```python
from build123d import *

# Parameters (mm, degrees)
SKETCH_1_R          = 3
EXTRUDE_1_DEPTH     = 1
SKETCH_2_R          = 2.5
EXTRUDE_2_DEPTH     = 7.6
FILLET_1_R          = 2.5
SKETCH_4_R          = 2.556662668
CUT_EXTRUDE_1_DEPTH = 1.1


with BuildPart() as part:
    # Эскиз1 → Бобышка-Вытянуть1 (new body)
    with BuildSketch(Plane(origin=(0, 0, 0), x_dir=(1, 0, 0), z_dir=(0, 1, 0))):
        with Locations(Location((0, 0, 0), (0, 0, 270))):
            Circle(SKETCH_1_R)
    extrude(amount=EXTRUDE_1_DEPTH)

    # Эскиз2 → Бобышка-Вытянуть2 (add)
    with BuildSketch(Plane(origin=(0, 1, 0), x_dir=(1, 0, 0), z_dir=(0, 1, 0))):
        with Locations(Location((0, 0, 0), (0, 0, 90))):
            Circle(SKETCH_2_R)
    extrude(amount=EXTRUDE_2_DEPTH)

    # Скругление1
    fillet_1_edges = [part.edges().sort_by_distance(p)[0] for p in [
        (0, 8.6, 2.5),
    ]]
    fillet(fillet_1_edges, radius=FILLET_1_R)

    # Эскиз4 → Вырез-Вытянуть1 (cut)
    with BuildSketch(Plane(origin=(0, 8.6, 0), x_dir=(1, 0, 0), z_dir=(0, 1, 0))):
        Circle(SKETCH_4_R)
    extrude(amount=-CUT_EXTRUDE_1_DEPTH, mode=Mode.SUBTRACT)


solid = part.part
```
For this review, take the finished solid that the model builds, in its own axes (mm). A direction names the side the tool comes from. Round coordinates to 2 decimals unless told otherwise and drop trailing zeros. Write each loop counter-clockwise with the first axis right and the second up, starting at its lowest first coordinate (ties: lowest second). Pieces come first, ordered by that corner, then holes. Notation, with made-up numbers: (43, 3) - (88, 3) arc R13 cw to (88, 26) - close; hole circle Ø9 at (-13, -26.75). An arc over 180 degrees is marked (long way). Answer as a JSON object with one key per item and string values.
1. We need section C-C on y = 2.25. Give the boundary of the cut face in (x, z).
Response values:
{"outline": "circle Ø5 at (0, 0)"}
2. For pin 1 Ø1 at (x, y) = (-1, 6.5) entering from +Z; pin 2 Ø1 at (y, z) = (2.5, 0) entering from +X; pin 3 Ø2 at (x, y) = (2, 4) entering from -Z, all flat-tipped, find the tip position at first contact; note any pin that passes through.
Response values:
{"pin 1": "stops at z = 2.43", "pin 2": "stops at x = 2.5", "pin 3": "stops at z = -2.29"}
3. To check wall thickness, follow line 1 along Y through (x, z) = (-2.3, 1.85); line 2 along Z through (x, y) = (0.05, 2). State the ranges of each line that lie inside material, in increasing order.
Response values:
{"line 1": "y = 0 to 1", "line 2": "z = -2.5 to 2.5"}
4. Tool access review of faces 1 (the face through (2.44, 3.51, 0.54)), 2 (the face through (0, 7.5, 0)): name each direction out of +Z, -Z, +X, -X, +Y, -Y from which nothing blocks a thin tool from reaching the whole face with its end or side.
Response values:
{"face 1": "+Y", "face 2": "+Z, -Z, +X, -X, +Y"}
5. We need section B-B on x = 0. Give the boundary of the cut face in (y, z), then the cut area to 3 significant figures.
Response values:
{"outline": "(0, -3) - (1, -3) - (1, -2.5) - (6.1, -2.5) arc R2.5 ccw to (7.5, -2.07) - (7.5, 2.07) arc R2.5 ccw to (6.1, 2.5) - (1, 2.5) - (1, 3) - (0, 3) - close", "area": "38.1 mm2"}
6. We need section A-A on z = 0. Give the boundary of the cut face in (x, y), then the cut area to 3 significant figures.
Response values:
{"outline": "(-3, 0) - (3, 0) - (3, 1) - (2.5, 1) - (2.5, 6.1) arc R2.5 ccw to (2.07, 7.5) - (-2.07, 7.5) arc R2.5 ccw to (-2.5, 6.1) - (-2.5, 1) - (-3, 1) - close", "area": "38.1 mm2"}
